```python
from build123d import *

# Parameters (mm, degrees)
SKETCH1_R           = 1.5
SKETCH1_R_2         = 10.5
SKETCH1_R_3         = 12
BOSS_EXTRUDE1_DEPTH = 5
SKETCH1_3_R         = 10.5
SKETCH1_3_R_2       = 9.5
BOSS_EXTRUDE2_DEPTH = 4


with BuildPart() as part:
    # Sketch1 → Boss-Extrude1 (new body)
    with BuildSketch(Plane.XY):
        with BuildLine():
            Line((60, 140), (25, 140))
            Line((25, 140), (-25, 75))
            Line((-25, 75), (-25, 0))
            Line((-25, 0), (50, 0))
            Line((50, 0), (60, 0))
            Line((60, 0), (60, 62.5))
            Line((60, 62.5), (80, 62.5))
            ThreePointArc((80, 62.5), (96.95996608, 71.9000212), (97.97752809, 91.264044944))
            Line((97.97752809, 91.264044944), (83.735955056, 120.47752809))
            ThreePointArc((83.735955056, 120.47752809), (79.12498675, 125.5999788), (72.5, 127.5))
            Line((72.5, 127.5), (60, 127.5))
            Line((60, 127.5), (60, 140))
        make_face()
        with Locations((-21.5, 9)):
            Circle(SKETCH1_R, mode=Mode.SUBTRACT)
        with Locations((-12.5, 62.5)):
            Circle(SKETCH1_R_2, mode=Mode.SUBTRACT)
        with Locations((56.5, 9)):
            Circle(SKETCH1_R, mode=Mode.SUBTRACT)
        with Locations((72, 68.643593539)):
            Circle(SKETCH1_R, mode=Mode.SUBTRACT)
        with Locations((88, 68.643593539)):
            Circle(SKETCH1_R, mode=Mode.SUBTRACT)
        with Locations((-16.867190649, 77.372042423)):
            Circle(SKETCH1_R, mode=Mode.SUBTRACT)
        with Locations((64, 82.5)):
            Circle(SKETCH1_R, mode=Mode.SUBTRACT)
        with Locations((80, 82.5)):
            Circle(SKETCH1_R_3, mode=Mode.SUBTRACT)
        with Locations((96, 82.5)):
            Circle(SKETCH1_R, mode=Mode.SUBTRACT)
        with Locations((72, 96.356406461)):
            Circle(SKETCH1_R, mode=Mode.SUBTRACT)
        with Locations((88, 96.356406461)):
            Circle(SKETCH1_R, mode=Mode.SUBTRACT)
        with Locations((56.5, 134)):
            Circle(SKETCH1_R, mode=Mode.SUBTRACT)
        with Locations((72.5, 115)):
            Circle(SKETCH1_R_2, mode=Mode.SUBTRACT)
    extrude(amount=BOSS_EXTRUDE1_DEPTH)

    # Sketch1_3 → Boss-Extrude2 (add)
    # profile 1 of 2: a face of its own
    with BuildSketch(Plane.XY):
        with Locations((-12.5, 62.5)):
            Circle(SKETCH1_3_R)
        with Locations((-12.5, 62.5)):
            Circle(SKETCH1_3_R_2, mode=Mode.SUBTRACT)
    # profile 2 of 2: a face of its own
    with BuildSketch(Plane.XY):
        with Locations((72.5, 115)):
            Circle(SKETCH1_3_R)
        with Locations((72.5, 115)):
            Circle(SKETCH1_3_R_2, mode=Mode.SUBTRACT)
    extrude(amount=BOSS_EXTRUDE2_DEPTH)


solid = part.part
```
Here's how the part is built. I have some questions about the finished solid (model axes, mm). A direction names the side the tool comes from. Coordinates: 2 decimals unless noted, no trailing zeros. Order: outer loops, then holes, each group sorted by start corner. A loop starts at its lowest first (then second) coordinate and runs counter-clockwise, first axis right, second up. Notation, with made-up numbers: M 28.5,40 L 52.5,40 A24 ccw 52.5,60 Z; hole C -2.75,-33 d3. An arc over 180 degrees is marked long. Answer as a JSON object with one key per item and string values. Group by question number.
(1) Suppose I cut it at D-D, the plane y = 31. Please give me the cut outline in (x, z), then the cut area to 3 significant figures.
(2) Which directions (+Z, -Z, +X, -X, +Y, -Y) give clear straight access to the entire face, cutting with the end or side of a thin tool? Please do faces 4 (the face through (57.306, 135.265, 2.465)), 5 (the face through (-15, 53, 4)).
(3) Suppose I cut it at A-A, the plane x = -12.5. Please give me the cut outline in (y, z), then the cut area to 3 significant figures.
(4) For pin 1 (2.5 mm diameter, centred on x = 65.5, z = 3, fed in from +Y); pin 2 (1.5 mm diameter, centred on y = 71.5, z = 4, fed in from +X), each with a flat end and sliding along its axis, tell me the tip position at first contact or that it passes through.
(5) I need wall thicknesses on probe 1 along X at (y, z) = (68, 3.7); probe 2 along Y at (x, z) = (65, 0.9); probe 3 along Y at (x, z) = (88, 2.95). Which ranges of each line are inside material? Lowest first, please.
(6) Suppose I cut it at B-B, the plane z = 1.85. State how many separate pieces and enclosed holes the cut face has, then the cut area to 3 significant figures.
(7) If we mould it in two halves opening along X, with no side actions, what happens to faces 1 (the face through (66, 127.5, 2)), 2 (the face through (70.22, 104.75, 4.49)), 3 (the face through (60, 31, 2))? For each: released by +X, released by -X, zero draft, split by the parting line, or undercut.
(8) Suppose I cut it at C-C, the plane y = 115. Please give me the cut outline in (x, z).
Values found:
{
 "1": {"outline": "M -25,0 L 60,0 L 60,5 L -25,5 Z", "area": "425 mm^2"},
 "2": {"face 4": "+Z, -Z", "face 5": "+Z"},
 "3": {"outline": "M 0,0 L 53,0 L 53,4 L 52,4 L 52,5 L 0,5 Z; M 72,0 L 91.25,0 L 91.25,5 L 73,5 L 73,4 L 72,4 Z", "area": "359 mm^2"},
 "4": {"pin 1": "stops at y = 127.5", "pin 2": "stops at x = 97.17"},
 "5": {"probe 1": "x = -25 to -20.25, -4.75 to 70.65, 73.35 to 86.65, 89.35 to 93.77", "probe 2": "y = 62.5 to 81.38, 83.62 to 109.17, 120.83 to 127.5", "probe 3": "y = 64.17 to 67.14, 70.14 to 73.56, 91.44 to 94.86, 97.86 to 111.73"},
 "6": {"separate pieces": "1", "enclosed holes": "13", "area": "11,300 mm^2"},
 "7": {"face 1": "zero draft", "face 2": "undercut", "face 3": "released by +X"},
 "8": {"outline": "M 5.77,0 L 63,0 L 63,4 L 62,4 L 62,5 L 5.77,5 Z; M 82,0 L 86.41,0 L 86.41,5 L 83,5 L 83,4 L 82,4 Z"}
}
